Read the model definition and answer for the solid it produces. Units are mm, in the model's axes. A direction names the side the tool comes from. Give positions to 0.01 mm unless a question says otherwise; leave off trailing zeros. Write each loop counter-clockwise with the first axis right and the second up, starting at its lowest first coordinate (ties: lowest second). Pieces come first, ordered by that corner, then holes. Notation, with made-up numbers: M 42,-16 L 95,-16 A19 ccw 95,7 Z; hole C 21,65.5 d3. An arc over 180 degrees is marked long. Put each result on its own line as item: value.
from build123d import *

# Parameters (mm, degrees)
SKETCH114_W               = 10
SKETCH114_H               = 10
F_40_X_40A_X_R0_5_1_DEPTH = 500


with BuildPart() as part:
    # Sketch114 → 铝型材 40 X 40A X R0.5(1) (new body)
    with BuildSketch(Plane.YX):
        with BuildLine():
            Line((-19.5, 20), (-4.5, 20))
            Line((-4.5, 20), (-4.5, 18.2))
            Line((-4.5, 18.2), (-7.1, 18.2))
            Line((-7.1, 18.2), (-7.1, 8.2))
            Line((-7.1, 8.2), (7.1, 8.2))
            Line((7.1, 8.2), (7.1, 18.2))
            Line((7.1, 18.2), (4.5, 18.2))
            Line((4.5, 18.2), (4.5, 20))
            Line((4.5, 20), (19.5, 20))
            ThreePointArc((19.5, 20), (19.853553391, 19.853553391), (20, 19.5))
            Line((20, 19.5), (20, 4.5))
            Line((20, 4.5), (18.2, 4.5))
            Line((18.2, 4.5), (18.2, 7.1))
            Line((18.2, 7.1), (8.2, 7.1))
            Line((8.2, 7.1), (8.2, -7.1))
            Line((8.2, -7.1), (18.2, -7.1))
            Line((18.2, -7.1), (18.2, -4.5))
            Line((18.2, -4.5), (20, -4.5))
            Line((20, -4.5), (20, -19.5))
            ThreePointArc((20, -19.5), (19.853553391, -19.853553391), (19.5, -20))
            Line((19.5, -20), (4.5, -20))
            Line((4.5, -20), (4.5, -18.2))
            Line((4.5, -18.2), (7.1, -18.2))
            Line((7.1, -18.2), (7.1, -8.2))
            Line((7.1, -8.2), (-7.1, -8.2))
            Line((-7.1, -8.2), (-7.1, -18.2))
            Line((-7.1, -18.2), (-4.5, -18.2))
            Line((-4.5, -18.2), (-4.5, -20))
            Line((-4.5, -20), (-19.5, -20))
            ThreePointArc((-19.5, -20), (-19.853553391, -19.853553391), (-20, -19.5))
            Line((-20, -19.5), (-20, -4.5))
            Line((-20, -4.5), (-18.2, -4.5))
            Line((-18.2, -4.5), (-18.2, -7.1))
            Line((-18.2, -7.1), (-8.2, -7.1))
            Line((-8.2, -7.1), (-8.2, 7.1))
            Line((-8.2, 7.1), (-18.2, 7.1))
            Line((-18.2, 7.1), (-18.2, 4.5))
            Line((-18.2, 4.5), (-20, 4.5))
            Line((-20, 4.5), (-20, 19.5))
            ThreePointArc((-20, 19.5), (-19.853553391, 19.853553391), (-19.5, 20))
        make_face()
        with BuildLine():
            Line((-4.87903679, 6.434671709), (-4.110433762, 5.66606868))
            ThreePointArc((-4.110433762, 5.66606868), (0, 7), (4.110433762, 5.66606868))
            Line((4.110433762, 5.66606868), (4.87903679, 6.434671709))
            ThreePointArc((4.87903679, 6.434671709), (6.434671709, 6.434671709), (6.434671709, 4.87903679))
            Line((6.434671709, 4.87903679), (5.66606868, 4.110433762))
            ThreePointArc((5.66606868, 4.110433762), (7, 0), (5.66606868, -4.110433762))
            Line((5.66606868, -4.110433762), (6.434671709, -4.87903679))
            ThreePointArc((6.434671709, -4.87903679), (6.434671709, -6.434671709), (4.87903679, -6.434671709))
            Line((4.87903679, -6.434671709), (4.110433762, -5.66606868))
            ThreePointArc((4.110433762, -5.66606868), (0, -7), (-4.110433762, -5.66606868))
            Line((-4.110433762, -5.66606868), (-4.87903679, -6.434671709))
            ThreePointArc((-4.87903679, -6.434671709), (-6.434671709, -6.434671709), (-6.434671709, -4.87903679))
            Line((-6.434671709, -4.87903679), (-5.66606868, -4.110433762))
            ThreePointArc((-5.66606868, -4.110433762), (-7, 0), (-5.66606868, 4.110433762))
            Line((-5.66606868, 4.110433762), (-6.434671709, 4.87903679))
            ThreePointArc((-6.434671709, 4.87903679), (-6.434671709, 6.434671709), (-4.87903679, 6.434671709))
        make_face(mode=Mode.SUBTRACT)
        with Locations((-13.7, 13.7)):
            Rectangle(SKETCH114_W, SKETCH114_H, mode=Mode.SUBTRACT)
        with Locations((13.7, 13.7)):
            Rectangle(SKETCH114_W, SKETCH114_H, mode=Mode.SUBTRACT)
        with Locations((13.7, -13.7)):
            Rectangle(SKETCH114_W, SKETCH114_H, mode=Mode.SUBTRACT)
        with Locations((-13.7, -13.7)):
            Rectangle(SKETCH114_W, SKETCH114_H, mode=Mode.SUBTRACT)
    extrude(amount=F_40_X_40A_X_R0_5_1_DEPTH)


solid = part.part
(1) For a pull along X with two mould halves and no side action, classify faces 1 (the face through (-12, 20, -246)), 2 (the face through (14, 8.7, -246)) as +X half, -X half, draft (parallel to the pull), parting line (faces both ways), or undercut.
Result:
face 1: draft
face 2: undercut
(2) Section B-B on z = -260.5 is taken. Give the number of separate pieces and of enclosed holes in the cut face, and give its area (3 significant figures).
Result:
separate pieces: 1
enclosed holes: 5
area: 396 mm²
(3) Section A-A on y = 13.5 is taken. Determine the outline of the cut face in (x, z).
Result:
outline: M -20,-500 L -18.7,-500 L -18.7,0 L -20,0 Z; M -8.7,-500 L -7.1,-500 L -7.1,0 L -8.7,0 Z; M 7.1,-500 L 8.7,-500 L 8.7,0 L 7.1,0 Z; M 18.7,-500 L 20,-500 L 20,0 L 18.7,0 Z
(4) Which of the six approach directions +Z, -Z, +X, -X, +Y, -Y give full straight-line access (tool end or side, diameter ignored) to faces 3 (the face through (8.2, 0, -246)), 4 (the face through (12, 20, -246))?
Result:
face 3: +Z, -Z
face 4: +Z, -Z, +X, -X, +Y
(5) Straight lines are drawn through the part: line 1 along Y through (x, z) = (18, -128.5); line 2 along Y through (x, z) = (18.5, -350). For each, find the intervals that lie inside material, in ascending order. Write a range as from..to.
Result:
line 1: y = -20..-18.7, -8.7..-7.1, 7.1..8.7, 18.7..20
line 2: y = -20..-18.7, -8.7..-4.5, 4.5..8.7, 18.7..20
